Here's how the part is built. I have some questions about the finished solid (model axes, mm). A direction names the side the tool comes from. Round coordinates to 2 decimals unless told otherwise and drop trailing zeros. Loops run counter-clockwise (first coordinate to the right, second up) from the corner with the lowest first, then second, coordinate; pieces in that order, holes last. Notation, with made-up numbers: (35, -10.5) - (84, -10.5) arc R30 cw to (84, 23.5) - close; hole circle Ø4 at (0, -18). An arc over 180 degrees is marked (long way). Answer as a JSON object with one key per item and string values. Group by question number.
1) If I drill on line 1 along Y through (x, z) = (-3.65, 10); line 2 along Z through (x, y) = (-3.6, 0), over which ranges is the centre line in solid material (lowest first)? Write a range as [from, to].
2) I want a section at D-D, the plane x = 6.75. Please give me the cut outline in (y, z).
3) I want a section at A-A, the plane y = 0. Please give me the cut outline in (x, z), then the cut area to 3 significant figures.
4) Will these pins go through, and if not, where does the flat tip stop? P1, Ø5, axis at x = 0, y = 0, coming from the +Z side; P2, Ø6, axis at x = 0, z = 10, coming from the -Y side.
5) If we mould it in two halves opening along X, with no side actions, what happens to faces 1 (the face through (0, 5, 20)), 2 (the face through (-3.247, 0.143, 6.07)), 3 (the face through (-10, 0, 10))? For each: pulls with the +X half, pulls with the -X half, needs draft (parallel to the pull), parting line crosses it, or undercut.
6) I want a section at B-B, the plane x = 0. Please give me the cut outline in (y, z), then the cut area to 3 significant figures.
7) Which directions (+Z, -Z, +X, -X, +Y, -Y) give clear straight access to the entire face, cutting with the end or side of a thin tool? Please do faces 4 (the face through (0, 5, 10)), 5 (the face through (-5, 0, 10)), 6 (the face through (-2.395, 2.197, 16.203)).
8) I want a section at C-C, the plane z = 6. Please give me the cut outline in (x, y), then the cut area to 3 significant figures.
from build123d import *

# Parameters (mm, degrees)
F0_W     = 20
F0_H     = 20
F1_DEPTH = 20
F2_R     = 3.25
F3_DEPTH = 15
F4_R     = 3.25
F5_DEPTH = 15
F6_R     = 3.25
F7_DEPTH = 15


with BuildPart() as f1:
    # F0 (on Top) → F1 (new body)
    with BuildSketch(Plane.XY):
        Rectangle(F0_W, F0_H)
    extrude(amount=F1_DEPTH)

    # F2 (on face) → F3 (cut)
    with BuildSketch(Plane.XY.offset(20)):
        Circle(F2_R)
    extrude(amount=-F3_DEPTH, mode=Mode.SUBTRACT)

    # F4 (on face) → F5 (cut)
    with BuildSketch(Plane.XZ.offset(10)):
        with Locations((0, 10)):
            Circle(F4_R)
    extrude(amount=-F5_DEPTH, mode=Mode.SUBTRACT)

    # F6 (on face) → F7 (cut)
    with BuildSketch(Plane.YZ.offset(10)):
        with Locations((0, 10)):
            Circle(F6_R)
    extrude(amount=-F7_DEPTH, mode=Mode.SUBTRACT)


solid = f1.part
Outcome:
{
 "1": {"line 1": "[-10, -3.25], [3.25, 10]", "line 2": "[0, 6.75], [13.25, 20]"},
 "2": {"outline": "(-10, 0) - (10, 0) - (10, 20) - (-10, 20) - close; hole circle Ø6.5 at (0, 10)"},
 "3": {"outline": "(-10, 0) - (10, 0) - (10, 6.75) - (3.25, 6.75) - (3.25, 5) - (-3.25, 5) - (-3.25, 6.75) - (-5, 6.75) - (-5, 13.25) - (-3.25, 13.25) - (-3.25, 20) - (-10, 20) - close; (3.25, 13.25) - (10, 13.25) - (10, 20) - (3.25, 20) - close", "area": "247 mm^2"},
 "4": {"P1": "z = 5", "P2": "y = 5"},
 "5": {"face 1": "needs draft", "face 2": "undercut", "face 3": "pulls with the -X half"},
 "6": {"outline": "(-10, 0) - (10, 0) - (10, 20) - (3.25, 20) - (3.25, 13.25) - (5, 13.25) - (5, 6.75) - (3.25, 6.75) - (3.25, 5) - (-3.25, 5) - (-3.25, 6.75) - (-10, 6.75) - close; (-10, 13.25) - (-3.25, 13.25) - (-3.25, 20) - (-10, 20) - close", "area": "247 mm^2"},
 "7": {"face 4": "-Y", "face 5": "+X", "face 6": "+Z"},
 "8": {"outline": "(-10, -10) - (10, -10) - (10, 10) - (-10, 10) - close; hole circle Ø6.5 at (0, 0)", "area": "367 mm^2"}
}
